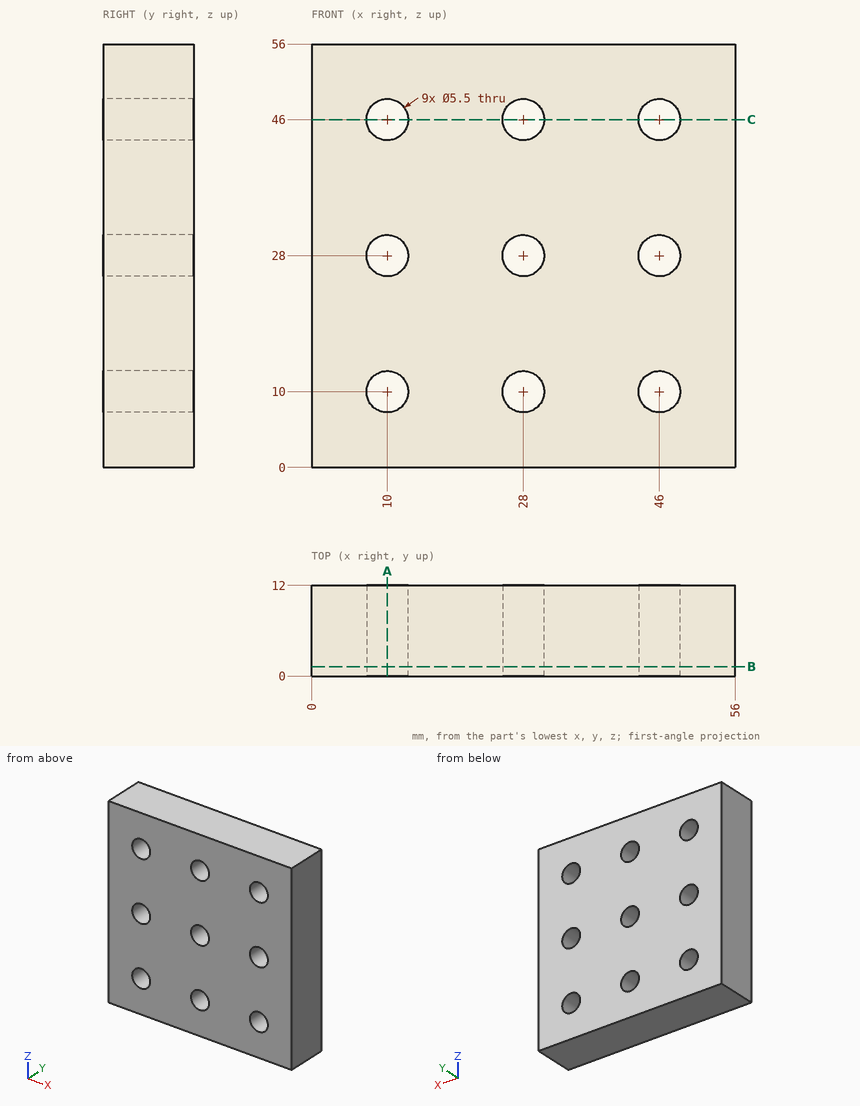
Can you work these out from the drawing? Everything is in mm from the part's minimum corner. Round coordinates to 2 decimals unless told otherwise and drop trailing zeros. Loops run counter-clockwise (first coordinate to the right, second up) from the corner with the lowest first, then second, coordinate; pieces in that order, holes last.
1. If I drill on line 1 along X through (y, z) = (11, 46); line 2 along X through (y, z) = (2.25, 47), over which ranges is the centre line in solid material (lowest first)?
Answer list:
line 1: x = 0 to 7.25, 12.75 to 25.25, 30.75 to 43.25, 48.75 to 56
line 2: x = 0 to 7.44, 12.56 to 25.44, 30.56 to 43.44, 48.56 to 56
2. If we section it at C-C on z = 46: Write out the boundary of the cut face in (x, y), plus the area to 3 significant figures.
Answer list:
outline: (0, 0) - (7.25, 0) - (7.25, 12) - (0, 12) - close; (12.75, 0) - (25.25, 0) - (25.25, 12) - (12.75, 12) - close; (30.75, 0) - (43.25, 0) - (43.25, 12) - (30.75, 12) - close; (48.75, 0) - (56, 0) - (56, 12) - (48.75, 12) - close
area: 474 mm2
3. If we section it at A-A on x = 10: Write out the boundary of the cut face in (y, z).
Answer list:
outline: (0, 0) - (12, 0) - (12, 7.25) - (0, 7.25) - close; (0, 12.75) - (12, 12.75) - (12, 25.25) - (0, 25.25) - close; (0, 30.75) - (12, 30.75) - (12, 43.25) - (0, 43.25) - close; (0, 48.75) - (12, 48.75) - (12, 56) - (0, 56) - close
4. If we section it at B-B on y = 1.25: Count the separate pieces of the cut face and the enclosed holes in it, plus the area to 3 significant figures.
Answer list:
separate pieces: 1
enclosed holes: 9
area: 2,920 mm2
